Geometry check sheet. Reference: the model listing, model coordinates, mm. A direction names the side the tool comes from. Round coordinates to 2 decimals unless told otherwise and drop trailing zeros. Write each loop counter-clockwise with the first axis right and the second up, starting at its lowest first coordinate (ties: lowest second). Pieces come first, ordered by that corner, then holes. Notation, with made-up numbers: (64.25, 46.25) -> (76.25, 46.25) arc R13 cw to (76.25, 69.25) -> close; hole circle Ø10 at (43, -21). An arc over 180 degrees is marked (long way). Use a Markdown table: item, result.
```python
from build123d import *

# Parameters (mm, degrees)
SKETCH_1_W          = 70
SKETCH_1_H          = 19.75
EXTRUDE_1_DEPTH     = 8
SKETCH_2_R          = 3
CUT_EXTRUDE_1_DEPTH = 9
SKETCH_9_R          = 1.5
CUT_EXTRUDE_7_DEPTH = 9
SKETCH_10_R         = 1.5
CUT_EXTRUDE_8_DEPTH = 20.75
FILLET_1_R          = 5
SKETCH_11_R         = 3.5
CUT_EXTRUDE_9_DEPTH = 2


with BuildPart() as part:
    # 草图1 → 凸台-拉伸1 (new body)
    with BuildSketch(Plane(origin=(0, 0, 0), x_dir=(1, 0, 0), z_dir=(0, 1, 0))):
        Rectangle(SKETCH_1_W, SKETCH_1_H)
    extrude(amount=EXTRUDE_1_DEPTH)

    # 草图2 → 切除-拉伸1 (cut, through all)
    with BuildSketch(Plane(origin=(0, 8, 0), x_dir=(1, 0, 0), z_dir=(0, 1, 0))):
        with Locations((-21.5, -0.125)):
            Circle(SKETCH_2_R)
        with Locations((21.5, -0.125)):
            Circle(SKETCH_2_R)
    extrude(amount=-CUT_EXTRUDE_1_DEPTH, mode=Mode.SUBTRACT)

    # 草图9 → 切除-拉伸7 (cut, through all)
    with BuildSketch(Plane(origin=(0, 8, 0), x_dir=(1, 0, 0), z_dir=(0, 1, 0))):
        with Locations((-15, 5.875)):
            Circle(SKETCH_9_R)
        with Locations((15, 5.875)):
            Circle(SKETCH_9_R)
    extrude(amount=-CUT_EXTRUDE_7_DEPTH, mode=Mode.SUBTRACT)

    # 草图10 → 切除-拉伸8 (cut, through all)
    with BuildSketch(Plane(origin=(0, 0, -9.875), x_dir=(-1, 0, 0), z_dir=(0, 0, -1))):
        with Locations((0, 4)):
            Circle(SKETCH_10_R)
    extrude(amount=-CUT_EXTRUDE_8_DEPTH, mode=Mode.SUBTRACT)

    # 圆角1
    fillet_1_edges = [part.edges().sort_by_distance(p)[0] for p in [
        (35, 4, 9.875),
        (-35, 4, 9.875),
        (-35, 4, -9.875),
        (35, 4, -9.875),
    ]]
    fillet(fillet_1_edges, radius=FILLET_1_R)

    # 草图11 → 切除-拉伸9 (cut)
    with BuildSketch(Plane(origin=(0, 0, -9.875), x_dir=(-1, 0, 0), z_dir=(0, 0, -1))):
        with Locations((0, 4)):
            Circle(SKETCH_11_R)
    extrude(amount=-CUT_EXTRUDE_9_DEPTH, mode=Mode.SUBTRACT)


solid = part.part
```
(1) Access from +Z, -Z, +X, -X, +Y, -Y to the whole of each face (thin tool, end or side, straight path). Record for faces 5 (the face through (0.759, 0.583, -8.889)), 6 (the face through (13.5, 4.1, -5.9)).
A:
| item | result |
|---|---|
| face 5 | -Z |
| face 6 | +Y, -Y |
(2) Section check D-D on x = 0. Record the cut outline in (y, z) (3 decimals), plus the area to 4 significant figures.
A:
| item | result |
|---|---|
| outline | (0, -9.875) -> (0.5, -9.875) -> (0.5, -7.875) -> (2.5, -7.875) -> (2.5, 9.875) -> (0, 9.875) -> close; (5.5, -7.875) -> (7.5, -7.875) -> (7.5, -9.875) -> (8, -9.875) -> (8, 9.875) -> (5.5, 9.875) -> close |
| area | 90.75 mm2 |
(3) Section check B-B on y = 4. Record the cut outline in (x, z) (3 decimals).
A:
| item | result |
|---|---|
| outline | (-35, -4.875) arc R5 ccw to (-30, -9.875) -> (-3.5, -9.875) -> (-3.5, -7.875) -> (-1.5, -7.875) -> (-1.5, 9.875) -> (-30, 9.875) arc R5 ccw to (-35, 4.875) -> close; (1.5, -7.875) -> (3.5, -7.875) -> (3.5, -9.875) -> (30, -9.875) arc R5 ccw to (35, -4.875) -> (35, 4.875) arc R5 ccw to (30, 9.875) -> (1.5, 9.875) -> close; hole circle Ø6 at (-21.5, 0.125); hole circle Ø3 at (-15, -5.875); hole circle Ø3 at (15, -5.875); hole circle Ø6 at (21.5, 0.125) |
(4) Section check C-C on z = 1.5. Record the cut outline in (x, y), plus the area to 3 significant figures.
A:
| item | result |
|---|---|
| outline | (-35, 0) -> (-24.17, 0) -> (-24.17, 8) -> (-35, 8) -> close; (-18.83, 0) -> (18.83, 0) -> (18.83, 8) -> (-18.83, 8) -> close; (24.17, 0) -> (35, 0) -> (35, 8) -> (24.17, 8) -> close; hole circle Ø3 at (0, 4) |
| area | 468 mm2 |
(5) Gauge pin test, flat ends, axial feed: pin 1 Ø2 at (x, y) = (-0.5, 5.5) entering from -Z (3 decimals); pin 2 Ø4 at (x, y) = (0, 4) entering from +Z (3 decimals). Record the tip position at first contact, or that the pin passes through.
A:
| item | result |
|---|---|
| pin 1 | stops at z = -7.875 |
| pin 2 | stops at z = 9.875 |
(6) Thickness scan on line 1 (Y direction, x = 0, z = -9.15); line 2 (Z direction, x = 15, y = 4) (3 decimals); line 3 (Y direction, x = 0, z = 4.75). Record the ranges inside material, lowest first.
A:
| item | result |
|---|---|
| line 1 | y = 0 to 0.5, 7.5 to 8 |
| line 2 | z = -9.875 to -7.375, -4.375 to 9.875 |
| line 3 | y = 0 to 2.5, 5.5 to 8 |
(7) Section check A-A on x = -15. Record the cut outline in (y, z) (3 decimals), plus the area to 3 significant figures.
A:
| item | result |
|---|---|
| outline | (0, -9.875) -> (8, -9.875) -> (8, -7.375) -> (0, -7.375) -> close; (0, -4.375) -> (8, -4.375) -> (8, 9.875) -> (0, 9.875) -> close |
| area | 134 mm2 |
(8) Release check for a two-part mould opening along Z. For faces 1 (the face through (0, 8, 0)), 2 (the face through (-24.497, 4.056, -0.007)), 3 (the face through (0, 2, 9.875)), 4 (the face through (18.503, 4.056, -0.007)) record: +Z half, -Z half, draft (parallel to the pull), parting line (faces both ways), or undercut.
A:
| item | result |
|---|---|
| face 1 | draft |
| face 2 | undercut |
| face 3 | +Z half |
| face 4 | undercut |
